from build123d import *
from build123d import SkipClean  # not in build123d's __all__

# Parameters (mm, degrees)
F0_W      = 80
F0_H      = 40
F1_DEPTH  = 12
F2_W      = 80
F2_H      = 10
F3_DEPTH  = 48
F6_DEPTH  = 30
F7_R      = 10
F8_DEPTH  = 282
F10_DEPTH = 25


# Not quite as in the source:
# - a feature names something its author has since deleted; it is built from what else it names


with BuildPart() as f1:
    # F0 (on Top) → F1 (new body)
    with BuildSketch(Plane.XY):
        with Locations((15.4384085536, -20.999699384)):
            Rectangle(F0_W, F0_H)
    extrude(amount=F1_DEPTH)

    # F2 (on face) → F3 (join)
    with BuildSketch(Plane.XY.offset(12)):
        with Locations((15.4384085536, -5.999699384)):
            Rectangle(F2_W, F2_H)
    extrude(amount=F3_DEPTH)

    # F5 (on face) → F6 (join)
    with BuildSketch(Plane(origin=(0, -0.999699384, 0), x_dir=(-1, 0, 0), z_dir=(0, 1, 0))):
        with BuildLine():
            ThreePointArc((4.5615914464, 40), (-1.2962728753, 54.1421355692), (-15.4384083992, 60))
            ThreePointArc((-15.4384083992, 60), (-29.5805441228, 54.1421356783), (-35.4384085536, 40))
            Line((-35.4384085536, 40), (-25.4384085536, 40))
            ThreePointArc((-25.4384085536, 40), (-15.4384085536, 50), (-5.4384085536, 40))
            Line((-5.4384085536, 40), (4.5615914464, 40))
        make_face()
        with BuildLine():
            Line((-25.4384085536, 40), (-5.4384085536, 40))
            ThreePointArc((-5.4384085536, 40), (-15.4384085536, 50), (-25.4384085536, 40))
        make_face()
        with BuildLine():
            ThreePointArc((-25.4384085536, 40), (-15.4384085536, 30), (-5.4384085536, 40))
            Line((-5.4384085536, 40), (-25.4384085536, 40))
        make_face()
        with BuildLine():
            ThreePointArc((-35.4384085536, 40), (-15.4384085536, 20), (4.5615914464, 40))
            Line((4.5615914464, 40), (-5.4384085536, 40))
            ThreePointArc((-5.4384085536, 40), (-15.4384085536, 30), (-25.4384085536, 40))
            Line((-25.4384085536, 40), (-35.4384085536, 40))
        make_face()
    extrude(amount=-F6_DEPTH)

    # F7 (on face) → F8 (cut)
    with BuildSketch(Plane.XZ.offset(30.999699384)):
        with Locations((15.4384085536, 40)):
            Circle(F7_R)
    extrude(amount=-F8_DEPTH, mode=Mode.SUBTRACT)

    # F9 (on face) → F10 (cut)
    with BuildSketch(Plane.XZ.offset(10.999699384)):
        Polygon((55.4384085536, 60), (26.7936958102, 60), (32.6127306701, 50.2490321416), (55.4384085536, 12), align=None)
        with BuildLine():
            Line((32.6127306701, 50.2490321416), (26.7936958102, 60))
            Line((26.7936958102, 60), (15.4384085536, 60))
            ThreePointArc((15.4384085536, 60), (25.3131074647, 57.392248889), (32.6127306701, 50.2490321416))
        make_face()
        with BuildLine():
            ThreePointArc((-1.7359137949, 50.2490317528), (5.5637094457, 57.3922487772), (15.4384085536, 60))
            Line((15.4384085536, 60), (4.083121297, 60))
            Line((4.083121297, 60), (-1.7359137949, 50.2490317528))
        make_face()
        Polygon((-1.7359137949, 50.2490317528), (4.083121297, 60), (-24.5615914464, 60), (-24.5615914464, 12), align=None)
    with SkipClean():  # cleaning this boolean's faces spoils the solid; the shape is the same uncleaned
        extrude(amount=-F10_DEPTH, mode=Mode.SUBTRACT)


solid = f1.part
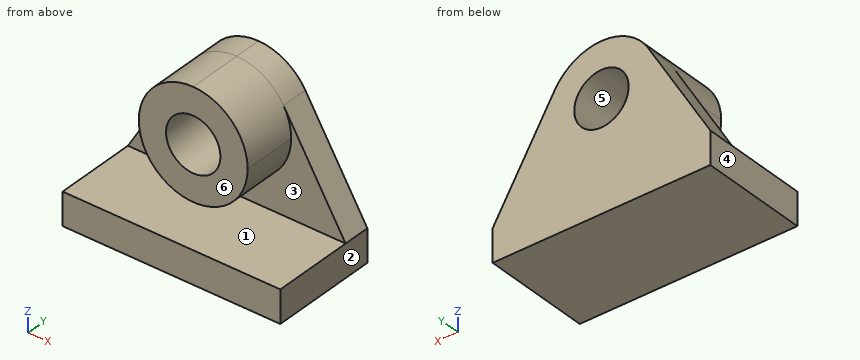
CAD build for the part. Positions are in the model's coordinates, mm. Face numbers are marked on the shaded views. A direction names the side the tool comes from. Round coordinates to 2 decimals unless told otherwise and drop trailing zeros. Order: outer loops, then holes, each group sorted by start corner. A loop starts at its lowest first (then second) coordinate and runs counter-clockwise, first axis right, second up. Notation, with made-up numbers: (68, -37) -> (72, -37) arc R16 ccw to (72, -17) -> close; hole circle Ø1 at (-8, -34.5). An arc over 180 degrees is marked (long way). Write item = value, one per line. Start each with the question number.
(1) Cut at A-A, the plane y = -29. List the corners of the cut face in (x, z).
(2) Probe line 1 (Z direction, x = 14, y = -18); line 2 (Y direction, x = 28.5, z = 32); line 3 (Y direction, x = 20, z = 17). List the from-to ranges inside material, lowest first. Write a range as [from, to].
(3) Cut at B-B, the plane z = 33. List the corners of the cut face in (x, y).
(4) Which spindle directions (+Z, -Z, +X, -X, +Y, -Y) get a long thin tool onto all of the face, cutting with end or side? Do the marked faces 1, 2 and 3. Say none if no direction does.
(5) Cut at D-D, the plane x = 41.5. List the corners of the cut face in (y, z).
(6) Pull direction X, two halves, no side cores. Call the marked faces 4, 5 and 6: released by +X, released by -X, zero draft, split by the parting line, or undercut.
(7) Pin check, flat tips, straight feed: P1, Ø2, axis at y = -5.5, z = 20.5, coming from the +X side; P2, Ø10, axis at y = -35, z = 30, coming from the -X side; P3, Ø1, axis at x = 22, y = -16, coming from the +Z side. Stop position of each tip, or through.
(8) Cut at C-C, the plane y = -9.5. List the corners of the cut face in (x, z).
Model answer:
q1.outline = (-24.56, 0) -> (55.44, 0) -> (55.44, 12) -> (-24.56, 12) -> close; circle Ø40 at (15.44, 40); hole circle Ø20 at (15.44, 40)
q2.line_1 = [0, 12], [20.05, 30.1], [49.9, 59.95]
q2.line_2 = [-31, -1]
q2.line_3 = [-11, -1]
q3.outline = (-12.03, -11) -> (-3.3, -11) -> (-3.3, -31) -> (8.3, -31) -> (8.3, -1) -> (-12.03, -1) -> close; (22.58, -31) -> (34.17, -31) -> (34.17, -11) -> (42.91, -11) -> (42.91, -1) -> (22.58, -1) -> close
q4.face_1 = +X, -X, -Y
q4.face_2 = +Z, -Z, +X, +Y, -Y
q4.face_3 = -Y
q5.outline = (-41, 0) -> (-1, 0) -> (-1, 35.36) -> (-11, 35.36) -> (-11, 12) -> (-41, 12) -> close
q6.face_4 = released by -X
q6.face_5 = undercut
q6.face_6 = zero draft
q7.P1 = 50.96
q7.P2 = -3.3
q7.P3 = 59.06
q8.outline = (-24.56, 0) -> (55.44, 0) -> (55.44, 12) -> (32.61, 50.25) arc R20 ccw to (-1.74, 50.25) -> (-24.56, 12) -> close; hole circle Ø20 at (15.44, 40)
